The listing builds one solid part. Answer for the finished solid, in the listing's coordinates (mm). Face numbers are marked on the shaded views. A direction names the side the tool comes from. Round coordinates to 2 decimals unless told otherwise and drop trailing zeros. Write each loop counter-clockwise with the first axis right and the second up, starting at its lowest first coordinate (ties: lowest second). Pieces come first, ordered by that corner, then holes.
from build123d import *

# Parameters (mm, degrees)
F0_W          = 30
F0_H          = 30
F1_DEPTH      = 42
F1_DEPTH_BACK = 7
F2_R          = 6.75
F3_DEPTH      = 15
F3_DEPTH_BACK = 7
F6_W          = 20
F6_H          = 25.0738771936
F7_DEPTH      = 5
F9_R          = 2.25
F10_DEPTH     = 50
F12_R         = 2.25
F13_DEPTH     = 7
F14_R         = 2.25
F15_DEPTH     = 14
F16_W         = 5
F16_H         = 5
F16_H_2       = 5.0838639587
F16_W_2       = 4.6232988685
F17_DEPTH     = 1
F18_R         = 1.5
F19_DEPTH     = 8.4197768095


with BuildPart() as f1:
    # F0 (on Top) → F1 (new body, two sides)
    with BuildSketch(Plane.XY) as f1_sk:
        Rectangle(F0_W, F0_H)
    extrude(amount=F1_DEPTH)
    extrude(f1_sk.sketch, amount=-F1_DEPTH_BACK)

    # F2 (on Top) → F3 (cut, two sides)
    with BuildSketch(Plane.XY) as f3_sk:
        Circle(F2_R)
    extrude(amount=F3_DEPTH, mode=Mode.SUBTRACT)
    extrude(f3_sk.sketch, amount=-F3_DEPTH_BACK, mode=Mode.SUBTRACT)

    # F6 (on face) → F7 (cut)
    with BuildSketch(Plane(origin=(0, -13.3626828422, 10.4400720362), x_dir=(-1, 0, 0), z_dir=(0, 0.7880107536, -0.6156614753))):
        with Locations((0, 21.5316948633)):
            Rectangle(F6_W, F6_H)
    extrude(amount=-F7_DEPTH, mode=Mode.SUBTRACT)

    # F9 (on offset) → F10 (cut)
    with BuildSketch(Plane.YZ.offset(15)):
        with Locations((-5.5286819115, 24.6767979115)):
            Circle(F9_R)
        with Locations((2.8317631222, 35.1947769523)):
            Circle(F9_R)
    extrude(amount=-F10_DEPTH, mode=Mode.SUBTRACT)

    # F12 (on offset) → F13 (cut)
    with BuildSketch(Plane.XZ.offset(15)):
        with Locations((0, 20.3330869851)):
            Circle(F12_R)
    extrude(amount=-F13_DEPTH, mode=Mode.SUBTRACT)

    # F14 (on offset) → F15 (cut)
    with BuildSketch(Plane.XZ.offset(15)):
        with Locations((0, 29.6528354788)):
            Circle(F14_R)
    extrude(amount=-F15_DEPTH, mode=Mode.SUBTRACT)

    # F16 (on face) → F17 (join)
    with BuildSketch(Plane.XY.offset(42)):
        with Locations((12.5, 12.5)):
            Rectangle(F16_W, F16_H)
        with Locations((12.5, -12.4580680206)):
            Rectangle(F16_W, F16_H_2)
        with Locations((-12.6883505657, -12.4580680206)):
            Rectangle(F16_W_2, F16_H_2)
        with Locations((-12.6883505657, 12.5)):
            Rectangle(F16_W_2, F16_H)
    extrude(amount=F17_DEPTH)

    # F18 (on face) → F19 (cut, through all)
    with BuildSketch(Plane.XZ.offset(15)):
        with Locations((0, 13)):
            Circle(F18_R)
    extrude(amount=-F19_DEPTH, mode=Mode.SUBTRACT)

    # F20 (on Right) → F21 (revolve, cut)
    with BuildSketch(Plane.YZ):
        Polygon((0, -7), (0, 0), (-10, -7), align=None)
    revolve(axis=Axis((0, 0, -3.5), (0, 0, -1)), mode=Mode.SUBTRACT)


solid = f1.part
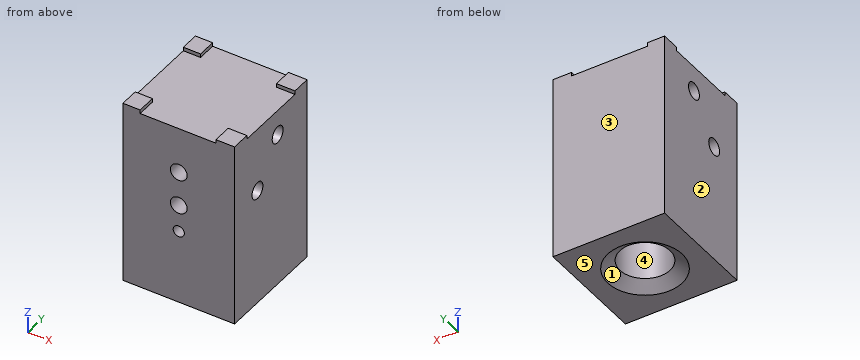
1. Section A-A on z = 13 is taken. Determine the outline of the cut face in (x, y), plus the area to 3 significant figures.
Geometry says:
outline: (-15, -15) - (-1.5, -15) - (-1.5, -6.58) arc R6.75 cw (long way) to (1.5, -6.58) - (1.5, -15) - (15, -15) - (15, 15) - (-15, 15) - close
area: 732 mm2
2. Given pin 1 (10 mm diameter, centred on x = -7.5, y = 0, fed in from +Z); pin 2 (5 mm diameter, centred on x = -5, y = 1.5, fed in from -Z), each flat-ended and moving along its own axis, determine where each tip first touches the part or whether it passes through.
Geometry says:
pin 1: stops at z = 42
pin 2: stops at z = -5.4
3. Section C-C on y = 0 is taken. Determine the outline of the cut face in (x, z) (3 decimals), plus the area to 3 significant figures.
Geometry says:
outline: (-15, -7) - (-10, -7) - (-6.75, -4.725) - (-6.75, 15) - (6.75, 15) - (6.75, -4.725) - (10, -7) - (15, -7) - (15, 42) - (-15, 42) - close; hole (-10, 27.544) - (10, 27.544) - (10, 35.665) - (-10, 35.665) - close
area: 1,000 mm2
4. Section B-B on x = 0 is taken. Determine the outline of the cut face in (y, z) (3 decimals), plus the area to 3 significant figures.
Geometry says:
outline: (-15, -7) - (-10, -7) - (-6.75, -4.725) - (-6.75, 11.5) - (-15, 11.5) - close; (-15, 14.5) - (-6.75, 14.5) - (-6.75, 15) - (6.75, 15) - (6.75, -4.725) - (10, -7) - (15, -7) - (15, 42) - (-15, 42) - (-15, 31.903) - (-2.939, 31.903) - (3.672, 40.365) - (7.612, 37.287) - (-7.825, 17.528) - (-8.535, 18.083) - (-15, 18.083) - close; (-15, 22.583) - (-10.221, 22.583) - (-6.455, 27.403) - (-15, 27.403) - close
area: 949 mm2
5. Section D-D on z = 5 is taken. Determine the outline of the cut face in (x, y).
Geometry says:
outline: (-15, -15) - (15, -15) - (15, 15) - (-15, 15) - close; hole circle Ø13.5 at (0, 0)
6. A tool of negligible diameter and unlimited length cuts with its end or side. For the marked faces 4 and 5, from which of +Z, -Z, +X, -X, +Y, -Y can it reach the whole face along a straight path? Write none if from no direction.
Geometry says:
face 4: -Z
face 5: -Z, +X, -X, +Y, -Y
7. Straight lines are drawn through the part: line 1 along Z through (x, y) = (0, -12.25); line 2 along X through (y, z) = (0, 7); line 3 along X through (y, z) = (-10, 13). For each, find the intervals that lie inside material, in ascending order.
Geometry says:
line 1: z = -7 to 11.5, 14.5 to 18.08, 22.58 to 27.4, 31.9 to 42
line 2: x = -15 to -6.75, 6.75 to 15
line 3: x = -15 to -1.5, 1.5 to 15
8. For a pull along X with two mould halves and no side action, classify the marked faces 1, 2 and 3 as released by +X, released by -X, zero draft, split by the parting line, or undercut.
Geometry says:
face 1: undercut
face 2: released by -X
face 3: zero draft
